Input: dimensioned drawing with shaded views. Units: mm. Origin: part minimum x, y, z. A direction names the side the tool comes from. Coordinates: 2 decimals unless noted, no trailing zeros. Order: outer loops, then holes, each group sorted by start corner. A loop starts at its lowest first (then second) coordinate and runs counter-clockwise, first axis right, second up. Notation, with made-up numbers: (29.25, -38) -> (68.25, -38) arc R18 ccw to (68.25, -33) -> close; hole circle Ø7 at (54.25, 3.5). An arc over 180 degrees is marked (long way). Answer in a Markdown table with one row per item. Add a question column.
1) Ray query, line 1 (Y direction, x = 4.5, z = 10); line 2 (Y direction, x = 11, z = 10). Return the intervals inside material, ascending. Write a range as from..to.
2) Section query D-D on y = 16. Return the cut outline in (x, z), then the cut area to 3 significant figures.
3) Contact query for flat-ended pins moving along their axis: P1, Ø6, axis at x = 4.5, y = 4, coming from the +Z side; P2, Ø7.5, axis at x = 12, z = 12.5, coming from the -Y side; P3, Ø3.5, axis at x = 10.5, z = 7.5, coming from the +Y side. Output: stop coordinate, or through.
4) Section query A-A on y = 10. Return the cut outline in (x, z).
5) Pull-direction query (Y, two-part tool) for the marked faces 3, 4, 5 and 6; classes: +Y half, -Y half, draft (parallel to the pull), parting line (faces both ways), or undercut.
6) Set-up query: the marked faces 1 and 2. Return all of +Z, -Z, +X, -X, +Y, -Y with unobstructed straight access to the full face (end or side cutting, diameter ignored); none if empty.
7) Section query C-C on x = 10.75. Return the cut outline in (y, z).
8) Section query B-B on z = 10. Return the cut outline in (x, y).
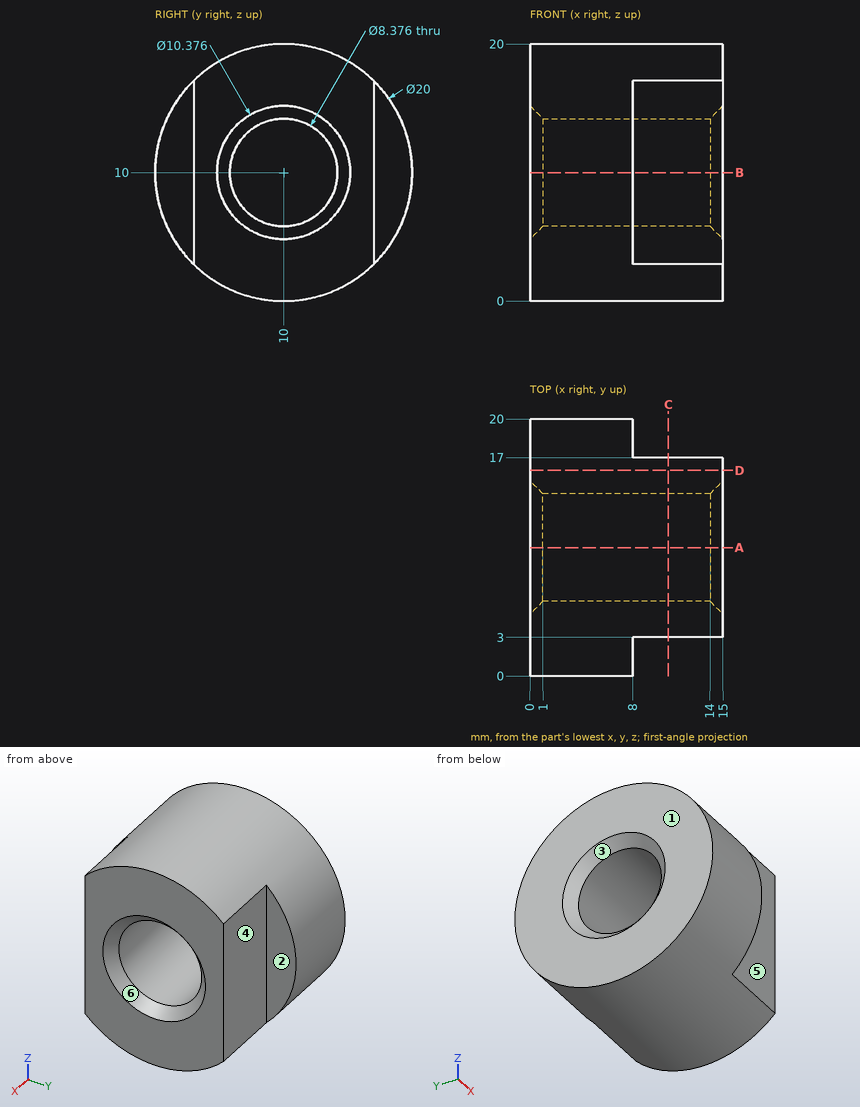
Result:
| question | item | result |
|---|---|---|
| 1 | line 1 | 0..5.81, 14.19..20 |
| 1 | line 2 | 3..5.81, 14.19..17 |
| 2 | outline | (0, 2) -> (15, 2) -> (15, 18) -> (0, 18) -> close |
| 2 | area | 240 mm2 |
| 3 | P1 | z = 19.54 |
| 3 | P2 | y = 3 |
| 3 | P3 | y = 17 |
| 4 | outline | (0, 0) -> (15, 0) -> (15, 4.81) -> (14, 5.81) -> (1, 5.81) -> (0, 4.81) -> close; (0, 15.19) -> (1, 14.19) -> (14, 14.19) -> (15, 15.19) -> (15, 20) -> (0, 20) -> close |
| 5 | face 3 | undercut |
| 5 | face 4 | +Y half |
| 5 | face 5 | -Y half |
| 5 | face 6 | undercut |
| 6 | face 1 | +Z, -Z, -X, +Y, -Y |
| 6 | face 2 | +Z, -Z, +X, +Y |
| 7 | outline | (3, 2.86) arc R10 ccw to (17, 2.86) -> (17, 17.14) arc R10 ccw to (3, 17.14) -> close; hole circle Ø8.38 at (10, 10) |
| 8 | outline | (0, 0) -> (8, 0) -> (8, 3) -> (15, 3) -> (15, 4.81) -> (14, 5.81) -> (1, 5.81) -> (0, 4.81) -> close; (0, 15.19) -> (1, 14.19) -> (14, 14.19) -> (15, 15.19) -> (15, 17) -> (8, 17) -> (8, 20) -> (0, 20) -> close |
